```python
from build123d import *

# Parameters (mm, degrees)
F0_R     = 10
F1_DEPTH = 25
F2_SIZE  = 1
F3_R     = 5
F4_DEPTH = 20
F5_SIZE  = 0.5
F6_R     = 1.6
F7_DEPTH = 45.001


with BuildPart() as f1:
    # F0 (on Top) → F1 (new body)
    with BuildSketch(Plane.XY):
        Circle(F0_R)
    extrude(amount=F1_DEPTH)

    # F2
    f2_edges = [f1.edges().sort_by_distance(p)[0] for p in [
        (-10, 0, 25),
    ]]
    chamfer(f2_edges, length=F2_SIZE)

    # F3 (on face) → F4 (join)
    with BuildSketch(Plane(origin=(0, 0, 0), x_dir=(1, 0, 0), z_dir=(0, 0, -1))):
        Circle(F3_R)
    extrude(amount=F4_DEPTH)

    # F5
    f5_edges = [f1.edges().sort_by_distance(p)[0] for p in [
        (-5, 0, -20),
    ]]
    chamfer(f5_edges, length=F5_SIZE)

    # F6 (on face) → F7 (cut, through all)
    with BuildSketch(Plane.XY.offset(25)):
        Circle(F6_R)
    extrude(amount=-F7_DEPTH, mode=Mode.SUBTRACT)


solid = f1.part
```
Read the model definition and answer for the solid it produces. Units are mm, in the model's axes. A direction names the side the tool comes from. Give positions to 0.01 mm unless a question says otherwise; leave off trailing zeros. Order: outer loops, then holes, each group sorted by start corner. A loop starts at its lowest first (then second) coordinate and runs counter-clockwise, first axis right, second up.
(1) For faces 1 (the cylindrical face through (-1.08, 4.88, -9.61)), 2 (the flat face through (0, -2, 25)), determine the directions among +Z, -Z, +X, -X, +Y, -Y from which every point of the face is accessible in a straight line to the end or side of a thin tool.
(2) Straight lines are drawn through the part: L1, parallel to Y at x = 0, z = 4; L2, parallel to Y at x = 0, z = -4; L3, parallel to Z at x = -5.25, y = -4.25. For each, find the intervals that lie inside material, in ascending order.
(3) Find section A-A (y = 0). Give the vertices of the cut face in (x, z), plus the area to 3 significant figures.
(4) Find section D-D (z = 2.5). Give the vertices of the cut face in (x, y), plus the area to 3 significant figures.
(5) For a pull along Y with two mould halves and no side action, classify faces 3 (the flat face through (-5, -2, 0)), 4 (the cylindrical face through (-2.17, -9.76, 11.83)), 5 (the cylindrical face through (-1.27, -0.97, 2.82)) as released by +Y, released by -Y, zero draft, split by the parting line, or undercut.
(6) Given pin 1 (1.5 mm diameter, centred on x = -1, z = 9.5, fed in from +Y); pin 2 (8 mm diameter, centred on x = 5, z = 3, fed in from +Y); pin 3 (6 mm diameter, centred on y = -6.5, z = 13.5, fed in from -X), each flat-ended and moving along its own axis, determine where each tip first touches the part or whether it passes through.
(7) Find section C-C (z = -9). Give the vertices of the cut face in (x, y), plus the area to 3 significant figures.
Result sheet:
1. face 1: -Z
1. face 2: +Z, +X, -X, +Y, -Y
2. L1: y = -10 to -1.6, 1.6 to 10
2. L2: y = -5 to -1.6, 1.6 to 5
2. L3: z = 0 to 25
3. outline: (-10, 0) - (-5, 0) - (-5, -19.5) - (-4.5, -20) - (-1.6, -20) - (-1.6, 25) - (-9, 25) - (-10, 24) - close; (1.6, -20) - (4.5, -20) - (5, -19.5) - (5, 0) - (10, 0) - (10, 24) - (9, 25) - (1.6, 25) - close
3. area: 555 mm2
4. outline: circle Ø20 at (0, 0); hole circle Ø3.2 at (0, 0)
4. area: 306 mm2
5. face 3: zero draft
5. face 4: split by the parting line
5. face 5: undercut
6. pin 1: stops at y = 10
6. pin 2: stops at y = 9.95
6. pin 3: stops at x = -9.37
7. outline: circle Ø10 at (0, 0); hole circle Ø3.2 at (0, 0)
7. area: 70.5 mm2
